Geometry: final body of the model. Coordinates: model frame, mm. Face numbers are marked on the shaded views. Give positions to 0.01 mm unless a question says otherwise; leave off trailing zeros. Order: outer loops, then holes, each group sorted by start corner. A loop starts at its lowest first (then second) coordinate and runs counter-clockwise, first axis right, second up. Notation, with made-up numbers: (-38.5, -14) - (-6.5, -14) arc R27 cw to (-6.5, 19) - close; hole circle Ø10 at (7.25, 15.25). An arc over 180 degrees is marked (long way). Put each result on its own line as item: value. Start each with the question number.
1. Mould query, pull axis Y, two halves, no side actions, for the marked faces 1 and 2. Classes: pulls with the +Y half, pulls with the -Y half, needs draft (parallel to the pull), parting line crosses it, or undercut.
2. Section C-C on x = 80. Return the cut outline in (y, z).
3. Ray query, line 1 along Z through (x, y) = (80, 3.1); line 2 along Z through (x, y) = (39.5, 3.75). Return the intervals inside material, ascending. Write a range as from..to.
4. Section A-A on z = -100. Return the cut outline in (x, y).
5. Section B-B on y = 3.6. Count the separate pieces of the cut face and the enclosed holes in it, plus the area to 3 significant figures.
Autodesk Inventor part; units mm, degrees
ref_plane "YZ Plane" through (0, 0, 0) normal (1, 0, 0) x (0, 1, 0)
ref_plane "XZ Plane" through (0, 0, 0) normal (0, 1, 0) x (-1, 0, 0)
ref_plane "XY Plane" through (0, 0, 0) normal (0, 0, 1) x (1, 0, 0)
sketch "Sketch1" plane through (0, 0, 0) normal (0, 1, 0) x (-1, 0, 0)
  line L0 (0, 0) -> (-120, 0)
  line L1 (-120, 0) -> (-120, -120)
  line L2 (-120, -120) -> (0, -120)
  line L3 (0, -120) -> (0, 0)
  circle A0 centre (-20, -20) radius 2.5
  circle A1 centre (-40, -20) radius 2.5
  circle A2 centre (-60, -20) radius 2.5
  circle A3 centre (-80, -20) radius 2.5
  circle A4 centre (-100, -20) radius 2.5
  circle A5 centre (-20, -40) radius 2.5
  circle A6 centre (-40, -40) radius 2.5
  circle A7 centre (-60, -40) radius 2.5
  circle A8 centre (-80, -40) radius 2.5
  circle A9 centre (-100, -40) radius 2.5
  circle A10 centre (-20, -60) radius 2.5
  circle A11 centre (-40, -60) radius 2.5
  circle A12 centre (-60, -60) radius 2.5
  circle A13 centre (-80, -60) radius 2.5
  circle A14 centre (-100, -60) radius 2.5
  circle A15 centre (-20, -80) radius 2.5
  circle A16 centre (-40, -80) radius 2.5
  circle A17 centre (-60, -80) radius 2.5
  circle A18 centre (-80, -80) radius 2.5
  circle A19 centre (-100, -80) radius 2.5
  circle A20 centre (-20, -100) radius 2.5
  circle A21 centre (-40, -100) radius 2.5
  circle A22 centre (-60, -100) radius 2.5
  circle A23 centre (-80, -100) radius 2.5
  circle A24 centre (-100, -100) radius 2.5
  dimension "d0" = 120
  dimension "d1" = 120
  dimension "d2" = 5
  dimension "d4" = 20
  dimension "d5" = 20
  dimension "d8" = 20
  dimension "d11" = 20
extrude "Extrusion1" add sketch "Sketch1" along normal blind 5
fillet "Fillet1" radius 5 4 edges at (0, 2.5, -120) (0, 2.5, 0) (120, 2.5, 0) (120, 2.5, -120)
properties part number "5x5x5 solder helper"
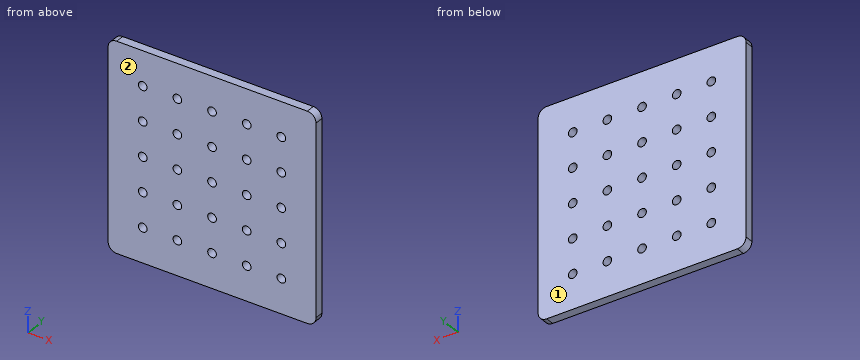
Resolved:
1. face 1: pulls with the +Y half
1. face 2: pulls with the -Y half
2. outline: (0, -120) - (5, -120) - (5, -102.5) - (0, -102.5) - close; (0, -97.5) - (5, -97.5) - (5, -82.5) - (0, -82.5) - close; (0, -77.5) - (5, -77.5) - (5, -62.5) - (0, -62.5) - close; (0, -57.5) - (5, -57.5) - (5, -42.5) - (0, -42.5) - close; (0, -37.5) - (5, -37.5) - (5, -22.5) - (0, -22.5) - close; (0, -17.5) - (5, -17.5) - (5, 0) - (0, 0) - close
3. line 1: -120..-102.5, -97.5..-82.5, -77.5..-62.5, -57.5..-42.5, -37.5..-22.5, -17.5..0
3. line 2: -120..-102.45, -97.55..-82.45, -77.55..-62.45, -57.55..-42.45, -37.55..-22.45, -17.55..0
4. outline: (0, 0) - (17.5, 0) - (17.5, 5) - (0, 5) - close; (22.5, 0) - (37.5, 0) - (37.5, 5) - (22.5, 5) - close; (42.5, 0) - (57.5, 0) - (57.5, 5) - (42.5, 5) - close; (62.5, 0) - (77.5, 0) - (77.5, 5) - (62.5, 5) - close; (82.5, 0) - (97.5, 0) - (97.5, 5) - (82.5, 5) - close; (102.5, 0) - (120, 0) - (120, 5) - (102.5, 5) - close
5. separate pieces: 1
5. enclosed holes: 25
5. area: 13,900 mm^2
